from build123d import *

# Parameters (mm, degrees)
F0_W      = 27
F0_H      = 15.9
F0_W_2    = 15.9
F0_H_2    = 27
F0_W_3    = 3
F0_H_3    = 3
F1_DEPTH  = 21.9
F2_DEPTH  = 51.8
F3_R      = 7.95
F6_DEPTH  = 30
F7_DEPTH  = 30
F4_R      = 7.9
F8_DEPTH  = 30
F10_W     = 4.4081552195
F10_H     = 4.2303893715
F11_DEPTH = 51.9
F13_DEPTH = 6.3
F14_W     = 19.4965768605
F14_H     = 3
F15_DEPTH = 26.1180568486
F16_R     = 1.5


with BuildPart() as f1:
    # F0 (on Front) → F1 (new body)
    with BuildSketch(Plane.XZ):
        with BuildLine():
            Line((-34.3576915575, 15.9), (-42.3076915575, 15.9))
            Line((-42.3076915575, 15.9), (-42.3076915575, 7.9499999931))
            ThreePointArc((-42.3076915575, 7.9499999931), (-39.9791904704, 13.571498908), (-34.3576915575, 15.9))
        make_face()
        with BuildLine():
            ThreePointArc((-34.3576915575, 15.9), (-39.9791904704, 13.571498908), (-42.3076915575, 7.9499999931))
            ThreePointArc((-42.3076915575, 7.9499999931), (-39.9791904655, 2.3285010871), (-34.3576915575, 0))
            ThreePointArc((-34.3576915575, 0), (-28.7361926471, 2.3285010896), (-26.4076915575, 7.95))
            ThreePointArc((-26.4076915575, 7.95), (-28.7361926471, 13.5714989104), (-34.3576915575, 15.9))
        make_face()
        Polygon((-42.3076915575, 18.9), (-42.3076915575, 45.9), (-26.4076915575, 45.9), (-26.4076915575, 18.9), (-23.4076915575, 18.9), (-23.4076915575, 48.9), (-45.3076915575, 48.9), (-45.3076915575, 18.9), align=None)
        with Locations((-9.9076915575, 7.95)):
            Rectangle(F0_W, F0_H)
        with Locations((-34.3576915575, 32.4)):
            Rectangle(F0_W_2, F0_H_2)
        with BuildLine():
            ThreePointArc((-34.3576915575, 0), (-39.9791904655, 2.3285010871), (-42.3076915575, 7.9499999931))
            Line((-42.3076915575, 7.9499999931), (-42.3076915575, 0))
            Line((-42.3076915575, 0), (-34.3576915575, 0))
        make_face()
        with BuildLine():
            Line((-26.4076915575, 0), (-26.4076915575, 7.95))
            ThreePointArc((-26.4076915575, 7.95), (-28.7361926471, 2.3285010896), (-34.3576915575, 0))
            Line((-34.3576915575, 0), (-26.4076915575, 0))
        make_face()
        with BuildLine():
            Line((-26.4076915575, 7.95), (-26.4076915575, 15.9))
            Line((-26.4076915575, 15.9), (-34.3576915575, 15.9))
            ThreePointArc((-34.3576915575, 15.9), (-28.7361926471, 13.5714989104), (-26.4076915575, 7.95))
        make_face()
        Polygon((6.5923084425, 18.9), (-23.4076915575, 18.9), (-23.4076915575, 15.9), (3.5923084425, 15.9), (3.5923084425, 0), (-23.4076915575, 0), (-23.4076915575, -3), (6.5923084425, -3), align=None)
        Polygon((-26.4076915575, 18.9), (-42.3076915575, 18.9), (-42.3076915575, 15.9), (-34.3576915575, 15.9), (-26.4076915575, 15.9), align=None)
        Polygon((-23.4076915575, 15.9), (-26.4076915575, 15.9), (-26.4076915575, 7.95), (-26.4076915575, 0), (-23.4076915575, 0), align=None)
        Polygon((-42.3076915575, 15.9), (-42.3076915575, 18.9), (-45.3076915575, 18.9), (-45.3076915575, -3), (-23.4076915575, -3), (-23.4076915575, 0), (-26.4076915575, 0), (-34.3576915575, 0), (-42.3076915575, 0), (-42.3076915575, 7.9499999931), align=None)
        with Locations((-24.9076915575, 17.4)):
            Rectangle(F0_W_3, F0_H_3)
    extrude(amount=F1_DEPTH)

    # F0 (on Front) → F2 (join)
    with BuildSketch(Plane.XZ):
        Polygon((-42.3076915575, 15.9), (-42.3076915575, 18.9), (-45.3076915575, 18.9), (-45.3076915575, -3), (-23.4076915575, -3), (-23.4076915575, 0), (-26.4076915575, 0), (-34.3576915575, 0), (-42.3076915575, 0), (-42.3076915575, 7.9499999931), align=None)
        with BuildLine():
            ThreePointArc((-34.3576915575, 15.9), (-39.9791904704, 13.571498908), (-42.3076915575, 7.9499999931))
            ThreePointArc((-42.3076915575, 7.9499999931), (-39.9791904655, 2.3285010871), (-34.3576915575, 0))
            ThreePointArc((-34.3576915575, 0), (-28.7361926471, 2.3285010896), (-26.4076915575, 7.95))
            ThreePointArc((-26.4076915575, 7.95), (-28.7361926471, 13.5714989104), (-34.3576915575, 15.9))
        make_face()
        Polygon((-26.4076915575, 18.9), (-42.3076915575, 18.9), (-42.3076915575, 15.9), (-34.3576915575, 15.9), (-26.4076915575, 15.9), align=None)
        Polygon((-23.4076915575, 15.9), (-26.4076915575, 15.9), (-26.4076915575, 7.95), (-26.4076915575, 0), (-23.4076915575, 0), align=None)
        with Locations((-24.9076915575, 17.4)):
            Rectangle(F0_W_3, F0_H_3)
        with BuildLine():
            Line((-26.4076915575, 7.95), (-26.4076915575, 15.9))
            Line((-26.4076915575, 15.9), (-34.3576915575, 15.9))
            ThreePointArc((-34.3576915575, 15.9), (-28.7361926471, 13.5714989104), (-26.4076915575, 7.95))
        make_face()
        with BuildLine():
            Line((-34.3576915575, 15.9), (-42.3076915575, 15.9))
            Line((-42.3076915575, 15.9), (-42.3076915575, 7.9499999931))
            ThreePointArc((-42.3076915575, 7.9499999931), (-39.9791904704, 13.571498908), (-34.3576915575, 15.9))
        make_face()
        with BuildLine():
            ThreePointArc((-34.3576915575, 0), (-39.9791904655, 2.3285010871), (-42.3076915575, 7.9499999931))
            Line((-42.3076915575, 7.9499999931), (-42.3076915575, 0))
            Line((-42.3076915575, 0), (-34.3576915575, 0))
        make_face()
        with BuildLine():
            Line((-26.4076915575, 0), (-26.4076915575, 7.95))
            ThreePointArc((-26.4076915575, 7.95), (-28.7361926471, 2.3285010896), (-34.3576915575, 0))
            Line((-34.3576915575, 0), (-26.4076915575, 0))
        make_face()
    extrude(amount=F2_DEPTH)

    # F3 (on face) → F6 (cut)
    with BuildSketch(Plane.XZ.offset(51.8)):
        with Locations((-34.3576915575, 7.95)):
            Circle(F3_R)
    extrude(amount=-F6_DEPTH, mode=Mode.SUBTRACT)

    # F5 (on face) → F7 (cut)
    with BuildSketch(Plane.YZ.offset(6.5923084425)):
        with BuildLine():
            ThreePointArc((-3, 7.95), (-5.3285010896, 13.5714989104), (-10.95, 15.9))
            ThreePointArc((-10.95, 15.9), (-16.5714989104, 13.5714989104), (-18.9, 7.95))
            ThreePointArc((-18.9, 7.95), (-16.5714989104, 2.3285010896), (-10.95, 0))
            ThreePointArc((-10.95, 0), (-5.3285010896, 2.3285010896), (-3, 7.95))
        make_face()
    extrude(amount=-F7_DEPTH, mode=Mode.SUBTRACT)

    # F4 (on face) → F8 (cut)
    with BuildSketch(Plane.XY.offset(48.9)):
        with Locations((-34.3576915575, -10.9)):
            Circle(F4_R)
    extrude(amount=-F8_DEPTH, mode=Mode.SUBTRACT)

    # F10 (on face) → F11 (join)
    with BuildSketch(Plane.XY.offset(48.9)):
        Polygon((-49.715846777, -11.3178612664), (-49.715846777, 3.9483262226), (-49.715846777, 8.1787155941), (-53.9462342858, 8.1787155941), (-53.9462342858, -11.3178612664), align=None)
        with Locations((-47.5117691672, 6.0635209084)):
            Rectangle(F10_W, F10_H)
        Polygon((-45.3076915575, 3.9483262226), (-45.3076915575, 0), (-39.9675555527, 0), (-39.9675555527, 3.9483262226), (-27.8281774372, 3.9483262226), (-27.8281774372, 8.1787155941), (-45.3076915575, 8.1787155941), align=None)
    extrude(amount=-F11_DEPTH)

    # F12 (on face) → F13 (join)
    with BuildSketch(Plane(origin=(0, 0, -3), x_dir=(1, 0, 0), z_dir=(0, 0, -1))):
        Polygon((-49.715846777, -8.1787155941), (-49.715846777, -3.9483262226), (-49.715846777, 11.3178612664), (-53.9462342858, 11.3178612664), (-53.9462342858, -8.1787155941), align=None)
    extrude(amount=F13_DEPTH)

    # F14 (on face) → F15 (join, through all)
    with BuildSketch(Plane(origin=(-53.9462342858, 0, 0), x_dir=(0, -1, 0), z_dir=(-1, 0, 0))):
        with Locations((1.5695728362, -7.8)):
            Rectangle(F14_W, F14_H)
    extrude(amount=-F15_DEPTH)

    # F16
    f16_edges = [f1.edges().sort_by_distance(p)[0] for p in [
        (-38.772012, 8.178716, -6.3),
        (-38.772012, 8.178716, -3),
        (-33.897866, 3.948326, 48.9),
        (-49.715847, -3.684768, 48.9),
        (-49.715847, 8.178716, -4.65),
    ]]
    fillet(f16_edges, radius=F16_R)


with BuildPart() as f17_1:
    # F17: instance of F1
    add(f1.part.mirror(Plane(origin=(6.5923084425, -10.95, 7.95), x_dir=(0, 1, 0), z_dir=(1, 0, 0))))


solid = f17_1.part
Work out the finished part from the listing and answer in its coordinate system (mm). A direction names the side the tool comes from. Round coordinates to 2 decimals unless told otherwise and drop trailing zeros. Loops run counter-clockwise (first coordinate to the right, second up) from the corner with the lowest first, then second, coordinate; pieces in that order, holes last. Notation, with made-up numbers: (-21.5, 39.5) - (7.5, 39.5) arc R21 cw to (7.5, 50.5) - close; hole circle Ø7 at (-36, 26.25). An arc over 180 degrees is marked (long way). Use one line per item in the form item = value. Start each with the question number.
(1) Find section B-B on y = -9. Determine the outline of the cut face in (x, z).
(2) Which of the six approach directions +Z, -Z, +X, -X, +Y, -Y give full straight-line access (tool end or side, diameter ignored) to faces 1 (the face through (48, -21.8, 8)), 2 (the face through (52, -2, -6.3)), 3 (the face through (35, 0, 18)), 4 (the face through (48, -11, 18.9)), 5 (the face through (48, -21.9, 34))?
(3) Find section A-A on z = 44.5. Determine the outline of the cut face in (x, y), and give its area (3 significant figures).
(4) Find section D-D on y = -43. Determine the outline of the cut face in (x, z), and give its area (3 significant figures).
(5) Flat-ended cylindrical pins translate along their axes: P1, Ø24, axis at x = 24, z = 11, coming from the -Y side; P2, Ø17.5, axis at y = -6.5, z = 32, coming from the -X side; P3, Ø2, axis at x = 60, z = 32, coming from the -Y side; P4, Ø20, axis at y = -2.5, z = 27, coming from the -X side. Find the tip coordinate at first contact, or state that the pin passes through.
(6) Find section C-C on x = 42. Determine the outline of the cut face in (y, z).
(7) Determine the mould class of faces 6 (the face through (53.152, 2, 23)), 7 (the face through (58.492, -17, 18)), 8 (the face through (52, -3, 48.9)) for opening direction X: +X half, -X half, draft (parallel to the pull), parting line (faces both ways), or undercut.
(8) Consider line 1 (Z direction, x = 46.5, y = -4); line 2 (X direction, y = 1.5, z = 22.5); line 3 (X direction, y = -43, z = 7). Determine where each line is inside the solid, lowest interval first.
Answer list:
q1.outline = (6.59, -3) - (58.49, -3) - (58.49, 48.9) - (55.21, 48.9) - (55.21, 18.9) - (39.87, 18.9) - (39.87, 48.9) - (36.59, 48.9) - (36.59, 18.9) - (6.59, 18.9) - (6.59, 15.66) - (36.59, 15.66) - (36.59, 0.24) - (6.59, 0.24) - close; (41.01, -9.3) - (67.13, -9.3) - (67.13, 48.9) - (64.4, 48.9) arc R1.5 ccw to (62.9, 47.4) - (62.9, -6.3) - (41.01, -6.3) - close
q2.face_1 = -Y
q2.face_2 = -X, +Y, -Y
q2.face_3 = +Z, -X
q2.face_4 = +Z
q2.face_5 = +Z, +X, -X, -Y
q3.outline = (36.59, -21.9) - (58.49, -21.9) - (58.49, 3.95) - (62.9, 3.95) - (62.9, -11.32) - (67.13, -11.32) - (67.13, 8.18) - (41.01, 8.18) - (41.01, 3.95) - (53.15, 3.95) - (53.15, 0) - (36.59, 0) - close; hole circle Ø15.8 at (47.54, -10.9)
q3.area = 480 mm^2
q4.outline = (36.59, -3) - (58.49, -3) - (58.49, 18.9) - (36.59, 18.9) - close; hole circle Ø15.9 at (47.54, 7.95)
q4.area = 281 mm^2
q5.P1 = -21.9
q5.P2 = 36.59
q5.P3 = 3.95
q5.P4 = 6.59
q6.outline = (-51.8, -3) - (0, -3) - (0, 48.9) - (-5.27, 48.9) - (-5.27, 18.9) - (-16.53, 18.9) - (-16.53, 48.9) - (-21.9, 48.9) - (-21.9, 18.9) - (-51.8, 18.9) - (-51.8, 13.65) - (-21.8, 13.65) - (-21.8, 2.25) - (-51.8, 2.25) - close; (-11.32, -9.3) - (8.18, -9.3) - (8.18, -7.8) arc R1.5 ccw to (6.68, -6.3) - (-11.32, -6.3) - close; (3.95, -3) - (6.68, -3) arc R1.5 ccw to (8.18, -1.5) - (8.18, 48.9) - (5.45, 48.9) arc R1.5 ccw to (3.95, 47.4) - close
q7.face_6 = -X half
q7.face_7 = undercut
q7.face_8 = draft
q8.line_1 = -9.3 to -6.3, -3 to 18.9
q8.line_2 = 53.15 to 58.49, 62.9 to 67.13
q8.line_3 = 36.59 to 39.65, 55.44 to 58.49
